from build123d import *

# Parameters (mm, degrees)
F0_W      = 63.5
F0_H      = 63.5
F1_DEPTH  = 44.45
F2_R      = 27.94
F3_DEPTH  = 5.08
F4_W      = 50.8
F4_H      = 19.05
F5_DEPTH  = 50.8
F7_R      = 1.905
F6_R      = 1.905
F8_DEPTH  = 1.27
F9_R      = 2.54
F10_W     = 2.54
F10_H     = 2.54
F11_DEPTH = 50.8


with BuildPart() as f1:
    # F0 (on Top) → F1 (new body)
    with BuildSketch(Plane.XY):
        Rectangle(F0_W, F0_H)
    extrude(amount=F1_DEPTH)

    # F2 (on face) → F3 (cut)
    with BuildSketch(Plane.XY.offset(44.45)):
        Circle(F2_R)
    extrude(amount=-F3_DEPTH, mode=Mode.SUBTRACT)

    # F4 (on face) → F5 (cut)
    with BuildSketch(Plane(origin=(-31.75, 0, 0), x_dir=(0, -1, 0), z_dir=(-1, 0, 0))):
        with Locations((0, 22.225)):
            Rectangle(F4_W, F4_H)
    extrude(amount=-F5_DEPTH, mode=Mode.SUBTRACT)

    # F7 (on face) + F6 (on face) → F8 (cut, symmetric)
    with BuildSketch(Plane(origin=(0, -25.4, 0), x_dir=(-1, 0, 0), z_dir=(0, 1, 0))):
        with Locations((29.21, 15.24)):
            Circle(F7_R)
    with BuildSketch(Plane.XZ.offset(-25.4)):
        with Locations((-29.21, 15.24)):
            Circle(F6_R)
    extrude(amount=F8_DEPTH, both=True, mode=Mode.SUBTRACT)

    # F9
    f9_edges = [f1.edges().sort_by_distance(p)[0] for p in [
        (0, 31.75, 44.45),
        (-31.75, 0, 44.45),
        (31.75, 0, 44.45),
        (0, -31.75, 44.45),
    ]]
    fillet(f9_edges, radius=F9_R)

    # F10 (on face) → F11 (join)
    with BuildSketch(Plane.XZ.offset(-25.4)):
        with Locations((-26.035, 30.226)):
            Rectangle(F10_W, F10_H)
    extrude(amount=F11_DEPTH)


solid = f1.part
Model file for the job. Use its own axes, mm. A direction names the side the tool comes from. Round coordinates to 2 decimals unless told otherwise and drop trailing zeros. Loops run counter-clockwise (first coordinate to the right, second up) from the corner with the lowest first, then second, coordinate; pieces in that order, holes last. Notation, with made-up numbers: (83.25, 5) - (114.25, 5) arc R17 cw to (114.25, 22) - close; hole circle Ø6 at (77.25, 16.25). An arc over 180 degrees is marked (long way). Write each question's results on one line, items separated by ' | '.
(1) Saw through at D-D, the plane z = 24. List the corners of the cut face in (x, y).
Answer below:
outline: (-31.75, -31.75) - (31.75, -31.75) - (31.75, 31.75) - (-31.75, 31.75) - (-31.75, 25.4) - (19.05, 25.4) - (19.05, -25.4) - (-31.75, -25.4) - close
(2) Mould opens along Z. For faces 6 (the cylindrical face through (-31.026, 0.444, 43.686)), 7 (the flat face through (0, -31.75, 21)), 8 (the flat face through (-29, -26.67, 15)) say: released by +Z, released by -Z, zero draft, split by the parting line, or undercut.
Answer below:
face 6: released by +Z | face 7: zero draft | face 8: undercut
(3) Saw through at C-C, the plane z = 30.5. List the corners of the cut face in (x, y) (3 decimals), then the cut area to 3 significant figures.
Answer below:
outline: (-31.75, -31.75) - (31.75, -31.75) - (31.75, 31.75) - (-31.75, 31.75) - (-31.75, 25.4) - (-27.305, 25.4) - (-27.305, -25.4) - (-31.75, -25.4) - close; hole (-24.765, -25.4) - (19.05, -25.4) - (19.05, 25.4) - (-24.765, 25.4) - close | area: 1,580 mm^2
(4) Wall check: L1, parallel to Z at x = -7, y = 2.5; L2, parallel to Z at x = -27, y = -14; L3, parallel to Y at x = -19, z = 21. Give the ranges that are in metal, low to high.
Answer below:
L1: z = 0 to 12.7, 31.75 to 39.37 | L2: z = 0 to 12.7, 28.96 to 31.5, 31.75 to 44.45 | L3: y = -31.75 to -25.4, 25.4 to 31.75
(5) 3-axis set-ups, long thin cutter, end or side, ignore diameter. For faces 1 (the cylindrical face through (-30.97, -26.03, 14.51)), 2 (the cylindrical face through (0.444, 30.986, 43.726)), 3 (the flat face through (-31.75, 0, 11)), 4 (the flat face through (-26, 0, 31.496)), 5 (the flat face through (0, 0, 39.37)): which of +Z, -Z, +X, -X, +Y, -Y reach the whole face in a straight line?
Answer below:
face 1: none | face 2: +Z, +X, -X, +Y | face 3: +Z, -Z, -X, +Y, -Y | face 4: -X | face 5: +Z
(6) Saw through at B-B, the plane x = 0. List the corners of the cut face in (y, z).
Answer below:
outline: (-31.75, 0) - (31.75, 0) - (31.75, 41.91) arc R2.54 ccw to (29.21, 44.45) - (27.94, 44.45) - (27.94, 39.37) - (-27.94, 39.37) - (-27.94, 44.45) - (-29.21, 44.45) arc R2.54 ccw to (-31.75, 41.91) - close; hole (-25.4, 12.7) - (25.4, 12.7) - (25.4, 31.75) - (-25.4, 31.75) - close
(7) Saw through at A-A, the plane y = 0. List the corners of the cut face in (x, z) (3 decimals).
Answer below:
outline: (-31.75, 0) - (31.75, 0) - (31.75, 41.91) arc R2.54 ccw to (29.21, 44.45) - (27.94, 44.45) - (27.94, 39.37) - (-27.94, 39.37) - (-27.94, 44.45) - (-29.21, 44.45) arc R2.54 ccw to (-31.75, 41.91) - (-31.75, 31.75) - (19.05, 31.75) - (19.05, 12.7) - (-31.75, 12.7) - close; (-27.305, 28.956) - (-24.765, 28.956) - (-24.765, 31.496) - (-27.305, 31.496) - close
(8) Pin check, flat tips, straight feed: pin 1 (2 mm diameter, centred on y = -2, z = 30, fed in from -X) (3 decimals); pin 2 (6 mm diameter, centred on y = 5, z = 21.5, fed in from -X); pin 3 (3 mm diameter, centred on x = 17, y = -13, fed in from +Z). Stop position of each tip, or through.
Answer below:
pin 1: stops at x = -27.305 | pin 2: stops at x = 19.05 | pin 3: stops at z = 39.37
